Source: three-view drawing plus pictorial views. Frame: mm from the lowest corner of the part. A direction names the side the tool comes from. Give positions to 0.01 mm unless a question says otherwise; leave off trailing zeros. Loops run counter-clockwise (first coordinate to the right, second up) from the corner with the lowest first, then second, coordinate; pieces in that order, holes last. Notation, with made-up numbers: (14.25, 6) - (43.25, 6) arc R29 cw to (43.25, 44) - close; hole circle Ø6 at (65, 86). An arc over 180 degrees is marked (long way). Answer in a Markdown table with one row per item.
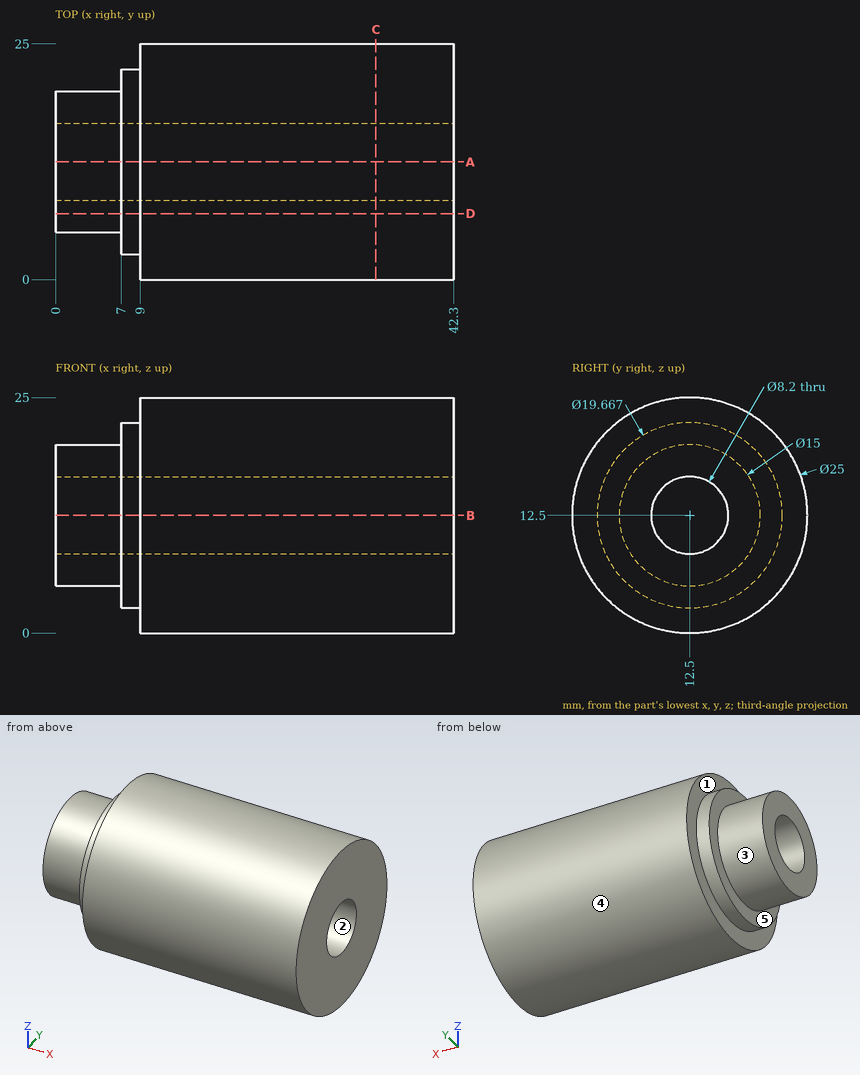
Q1. Cut plane A-A (y = 12.5). Output: boundary loops of the cut face in (x, z), and give its area (3 significant figures).
Check values:
| item | result |
|---|---|
| outline | (0, 5) - (7, 5) - (7, 2.67) - (9, 2.67) - (9, 0) - (42.3, 0) - (42.3, 8.4) - (0, 8.4) - close; (0, 16.6) - (42.3, 16.6) - (42.3, 25) - (9, 25) - (9, 22.33) - (7, 22.33) - (7, 20) - (0, 20) - close |
| area | 630 mm² |
Q2. Cut plane C-C (x = 34). Output: boundary loops of the cut face in (y, z), and give its area (3 significant figures).
Check values:
| item | result |
|---|---|
| outline | circle Ø25 at (12.5, 12.5); hole circle Ø8.2 at (12.5, 12.5) |
| area | 438 mm² |
Q3. First-contact query: pin 1 (10.5 mm diameter, centred on y = 12.5, z = 12.5, fed in from -X); pin 2 (5 mm diameter, centred on x = 8, z = 18.5, fed in from +Y); pin 3 (8 mm diameter, centred on x = 28, y = 4, fed in from -Z); pin 4 (3 mm diameter, centred on x = 21.5, y = 3.5, fed in from -Z). Flat tips, straight axial feed; report the tip coordinate or a pass-through.
Check values:
| item | result |
|---|---|
| pin 1 | x = 0 |
| pin 2 | y = 24.44 |
| pin 3 | z = 0.84 |
| pin 4 | z = 2.5 |
Q4. Cut plane D-D (y = 7). Output: boundary loops of the cut face in (x, z) (1 decimal).
Check values:
| item | result |
|---|---|
| outline | (0, 7.4) - (7, 7.4) - (7, 4.3) - (9, 4.3) - (9, 1.3) - (42.3, 1.3) - (42.3, 23.7) - (9, 23.7) - (9, 20.7) - (7, 20.7) - (7, 17.6) - (0, 17.6) - close |
Q5. Material intervals for line 1 along X through (y, z) = (19.75, 4.75); line 2 along Z through (x, y) = (6, 13); line 3 along X through (y, z) = (17, 20.25), sorted ascending.
Check values:
| item | result |
|---|---|
| line 1 | 9 to 42.3 |
| line 2 | 5.02 to 8.43, 16.57 to 19.98 |
| line 3 | 7 to 42.3 |
Q6. Draft query along Z for the marked faces 1, 2 and 3. Return one class per face: pulls with the +Z half, pulls with the -Z half, needs draft (parallel to the pull), parting line crosses it, or undercut.
Check values:
| item | result |
|---|---|
| face 1 | needs draft |
| face 2 | undercut |
| face 3 | parting line crosses it |
Q7. Reachability of the marked faces 4 and 5 from +Z, -Z, +X, -X, +Y, -Y: full face, straight path, thin tool, end or side. Return the list, or none.
Check values:
| item | result |
|---|---|
| face 4 | +X, -X |
| face 5 | -X |
